Part model, mm, in its own coordinate system. Give positions to 0.01 mm unless a question says otherwise; leave off trailing zeros. Loops run counter-clockwise (first coordinate to the right, second up) from the corner with the lowest first, then second, coordinate; pieces in that order, holes last. Notation, with made-up numbers: (38.25, 68.5) -> (46.25, 68.5) arc R8 cw to (46.25, 78.5) -> close; hole circle Ø6 at (-9, 74). An arc over 180 degrees is marked (long way). Write item = value, one per line.
from build123d import *

# Parameters (mm, degrees)
SKETCH1_W           = 25.4
SKETCH1_H           = 50.8
SKETCH1_W_2         = 19.05
SKETCH1_H_2         = 44.45
BOSS_EXTRUDE1_DEPTH = 965.2
SKETCH2_R           = 2.4892
CUT_EXTRUDE1_DEPTH  = 967.619351141


with BuildPart() as part:
    # Sketch1 → Boss-Extrude1 (new body)
    with BuildSketch(Plane.XY):
        Rectangle(SKETCH1_W, SKETCH1_H)
        Rectangle(SKETCH1_W_2, SKETCH1_H_2, mode=Mode.SUBTRACT)
    extrude(amount=BOSS_EXTRUDE1_DEPTH)

    # Sketch2 → Cut-Extrude1 (cut, through all)
    with BuildSketch(Plane(origin=(0, 25.4, 0), x_dir=(1, 0, 0), z_dir=(0, 1, 0))):
        with Locations(Location((0, -12.7, 0), (0, 0, 270))):
            Circle(SKETCH2_R)
        with Locations(Location((0, -38.1, 0), (0, 0, 270))):
            Circle(SKETCH2_R)
        with Locations(Location((0, -63.5, 0), (0, 0, 270))):
            Circle(SKETCH2_R)
        with Locations(Location((0, -88.9, 0), (0, 0, 270))):
            Circle(SKETCH2_R)
        with Locations(Location((0, -114.3, 0), (0, 0, 270))):
            Circle(SKETCH2_R)
        with Locations(Location((0, -139.7, 0), (0, 0, 270))):
            Circle(SKETCH2_R)
        with Locations(Location((0, -165.1, 0), (0, 0, 270))):
            Circle(SKETCH2_R)
        with Locations(Location((0, -190.5, 0), (0, 0, 270))):
            Circle(SKETCH2_R)
        with Locations(Location((0, -215.9, 0), (0, 0, 270))):
            Circle(SKETCH2_R)
        with Locations(Location((0, -241.3, 0), (0, 0, 270))):
            Circle(SKETCH2_R)
        with Locations(Location((0, -266.7, 0), (0, 0, 270))):
            Circle(SKETCH2_R)
        with Locations(Location((0, -292.1, 0), (0, 0, 270))):
            Circle(SKETCH2_R)
        with Locations(Location((0, -317.5, 0), (0, 0, 270))):
            Circle(SKETCH2_R)
        with Locations(Location((0, -342.9, 0), (0, 0, 270))):
            Circle(SKETCH2_R)
        with Locations(Location((0, -368.3, 0), (0, 0, 270))):
            Circle(SKETCH2_R)
        with Locations(Location((0, -393.7, 0), (0, 0, 270))):
            Circle(SKETCH2_R)
        with Locations(Location((0, -419.1, 0), (0, 0, 270))):
            Circle(SKETCH2_R)
        with Locations(Location((0, -444.5, 0), (0, 0, 270))):
            Circle(SKETCH2_R)
        with Locations(Location((0, -469.9, 0), (0, 0, 270))):
            Circle(SKETCH2_R)
        with Locations(Location((0, -495.3, 0), (0, 0, 270))):
            Circle(SKETCH2_R)
        with Locations(Location((0, -520.7, 0), (0, 0, 270))):
            Circle(SKETCH2_R)
        with Locations(Location((0, -546.1, 0), (0, 0, 270))):
            Circle(SKETCH2_R)
        with Locations(Location((0, -571.5, 0), (0, 0, 270))):
            Circle(SKETCH2_R)
        with Locations(Location((0, -596.9, 0), (0, 0, 270))):
            Circle(SKETCH2_R)
        with Locations(Location((0, -622.3, 0), (0, 0, 270))):
            Circle(SKETCH2_R)
        with Locations(Location((0, -647.7, 0), (0, 0, 270))):
            Circle(SKETCH2_R)
        with Locations(Location((0, -673.1, 0), (0, 0, 270))):
            Circle(SKETCH2_R)
        with Locations(Location((0, -698.5, 0), (0, 0, 270))):
            Circle(SKETCH2_R)
        with Locations(Location((0, -723.9, 0), (0, 0, 270))):
            Circle(SKETCH2_R)
        with Locations(Location((0, -749.3, 0), (0, 0, 270))):
            Circle(SKETCH2_R)
        with Locations(Location((0, -774.7, 0), (0, 0, 270))):
            Circle(SKETCH2_R)
        with Locations(Location((0, -800.1, 0), (0, 0, 270))):
            Circle(SKETCH2_R)
        with Locations(Location((0, -825.5, 0), (0, 0, 270))):
            Circle(SKETCH2_R)
        with Locations(Location((0, -850.9, 0), (0, 0, 270))):
            Circle(SKETCH2_R)
        with Locations(Location((0, -876.3, 0), (0, 0, 270))):
            Circle(SKETCH2_R)
        with Locations(Location((0, -901.7, 0), (0, 0, 270))):
            Circle(SKETCH2_R)
        with Locations(Location((0, -927.1, 0), (0, 0, 270))):
            Circle(SKETCH2_R)
        with Locations(Location((0, -952.5, 0), (0, 0, 270))):
            Circle(SKETCH2_R)
        with Locations(Location((0, -76.2, 0), (0, 0, 270))):
            Circle(SKETCH2_R)
    extrude(amount=-CUT_EXTRUDE1_DEPTH, mode=Mode.SUBTRACT)


solid = part.part
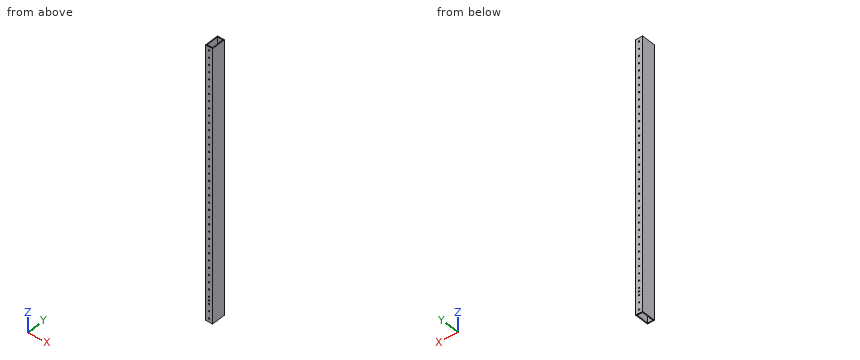
1) Drill centre lines: line 1 along Y through (x, z) = (-3, 844) (3 decimals); line 2 along X through (y, z) = (-5.5, 672.5) (3 decimals); line 3 along X through (y, z) = (-23, 723). Where is each one in solid material? Low to high. Write a range as [from, to].
Resolved:
line_1 = [-25.4, -22.225], [22.225, 25.4]
line_2 = [-12.7, -9.525], [9.525, 12.7]
line_3 = [-12.7, -2.32], [2.32, 12.7]
2) Drop a flat-ended pin along its axis: P1, Ø4, axis at x = 0, z = 850.9, coming from the +Y side. Give the stop position or say it passes through.
Resolved:
P1 = through
3) Slice it at B-B, the plane z = 662. List the corners of the cut face in (x, y) (3 decimals).
Resolved:
outline = (-12.7, -25.4) -> (12.7, -25.4) -> (12.7, 25.4) -> (-12.7, 25.4) -> close; hole (-9.525, -22.225) -> (9.525, -22.225) -> (9.525, 22.225) -> (-9.525, 22.225) -> close
4) Slice it at A-A, the plane y = -6. List the corners of the cut face in (x, z) (3 decimals), and give its area (3 significant figures).
Resolved:
outline = (-12.7, 0) -> (-9.525, 0) -> (-9.525, 965.2) -> (-12.7, 965.2) -> close; (9.525, 0) -> (12.7, 0) -> (12.7, 965.2) -> (9.525, 965.2) -> close
area = 6,130 mm²
